Input: part model. Units: mm. Frame: model coordinates. A direction names the side the tool comes from. Coordinates: 2 decimals unless noted, no trailing zeros. Write each loop counter-clockwise with the first axis right and the second up, starting at its lowest first coordinate (ties: lowest second). Pieces come first, ordered by that corner, then holes. Notation, with made-up numbers: (55.5, 10) - (77.5, 10) arc R31 ccw to (77.5, 49) - close; hole circle Ø10 at (66.25, 30). An arc over 180 degrees is marked (long way). Use CSV: the item, a comma, the result in double quotes.
```python
from build123d import *

# Parameters (mm, degrees)
F2_R     = 2.38125
F3_DEPTH = 12.7
F4_R     = 5.715
F5_DEPTH = 12.7


with BuildPart() as f1:
    # F0 (on Front) → F1 (revolve)
    with BuildSketch(Plane.XZ):
        Polygon((0, -1.2290018785), (0, 11.6460951906), (-9.525, 11.6460951906), (-9.525, 2.1210951906), (-11.1125, 2.1210951906), (-11.1125, 0), (-9.525, -0.637396297), (-4.7625, -1.2290018785), align=None)
    revolve(axis=Axis((0, 0, 5.2085466561), (0, 0, -1)))

    # F2 (on Front) → F3 (cut, symmetric)
    with BuildSketch(Plane.XZ):
        with Locations((0, 6.8835951906)):
            Circle(F2_R)
    extrude(amount=F3_DEPTH, both=True, mode=Mode.SUBTRACT)

    # F4 (on Top) → F5 (cut, symmetric)
    with BuildSketch(Plane.XY):
        Circle(F4_R)
    extrude(amount=F5_DEPTH, both=True, mode=Mode.SUBTRACT)


solid = f1.part
```
(1) Cut plane A-A on x = 0. Return loops of the section in (y, z) (1 decimal).
Check values:
outline,"(-11.1, 0) - (-9.5, -0.6) - (-5.7, -1.1) - (-5.7, 4.5) - (-9.5, 4.5) - (-9.5, 2.1) - (-11.1, 2.1) - close; (-9.5, 9.3) - (-5.7, 9.3) - (-5.7, 11.6) - (-9.5, 11.6) - close; (5.7, -1.1) - (9.5, -0.6) - (11.1, 0) - (11.1, 2.1) - (9.5, 2.1) - (9.5, 4.5) - (5.7, 4.5) - close; (5.7, 9.3) - (9.5, 9.3) - (9.5, 11.6) - (5.7, 11.6) - close"
(2) Cut plane C-C on z = 7.25. Return loops of the section in (x, y) (3 decimals), and give its area (3 significant figures).
Check values:
outline,"(-2.353, -9.23) - (-2.353, -5.208) arc R5.715 cw to (-2.353, 5.208) - (-2.353, 9.23) arc R9.525 ccw to start; (2.353, -9.23) arc R9.525 ccw to (2.353, 9.23) - (2.353, 5.208) arc R5.715 cw to (2.353, -5.208) - close"
area,"146 mm^2"
(3) Draft query along Z for faces 1 (the conical face through (4.682, -3.59, -1.088)), 2 (the flat face through (0, -6, 11.646)), 3 (the cylindrical face through (-2.38, -7.39, 6.99)). Return one class per face: pulls with the +Z half, pulls with the -Z half, needs draft (parallel to the pull), parting line crosses it, or undercut.
Check values:
face 1,"pulls with the -Z half"
face 2,"pulls with the +Z half"
face 3,"undercut"
(4) Cut plane D-D on z = 2.75. Return loops of the section in (x, y) (3 decimals).
Check values:
outline,"circle Ø19.05 at (0, 0); hole circle Ø11.43 at (0, 0)"
(5) Ray query, probe 1 along Y at (x, z) = (0, 3) (3 decimals); probe 2 along X at (y, z) = (0.25, 1); probe 3 along X at (y, z) = (0, -0.25) (3 decimals). Return the intervals inside material, ascending. Write a range as from..to.
Check values:
probe 1,"-9.525..-5.715, 5.715..9.525"
probe 2,"-11.11..-5.71, 5.71..11.11"
probe 3,"-10.49..-5.715, 5.715..10.49"
(6) Pin query (flat end, axial travel): pin 1 Ø3 at (y, z) = (-3, 8) entering from -X; pin 2 Ø6 at (x, z) = (0, 6.88) entering from +Y (3 decimals); pin 3 Ø5 at (y, z) = (-6, 4) entering from +X. Return the tip coordinate at first contact, or that it passes through.
Check values:
pin 1,"x = -9.41"
pin 2,"y = 9.525"
pin 3,"x = 10.23"
(7) Cut plane B-B on y = 0. Return loops of the section in (x, z) (1 decimal), and give its area (3 significant figures).
Check values:
outline,"(-11.1, 0) - (-9.5, -0.6) - (-5.7, -1.1) - (-5.7, 11.6) - (-9.5, 11.6) - (-9.5, 2.1) - (-11.1, 2.1) - close; (5.7, -1.1) - (9.5, -0.6) - (11.1, 0) - (11.1, 2.1) - (9.5, 2.1) - (9.5, 11.6) - (5.7, 11.6) - close"
area,"103 mm^2"
(8) Reachability of faces 4 (the flat face through (-5, 8.3, 2.121)), 5 (the cylindrical face through (-0.52, 7.33, 4.56)) from +Z, -Z, +X, -X, +Y, -Y: full face, straight path, thin tool, end or side. Return the list, or none.
Check values:
face 4,"+Z"
face 5,"+Y, -Y"
